The figure shows three views and two pictorial views of one solid part (mm, origin at its lowest corner). Answer the questions. Round coordinates to 2 decimals unless told otherwise and drop trailing zeros. Write each loop counter-clockwise with the first axis right and the second up, starting at its lowest first coordinate (ties: lowest second). Pieces come first, ordered by that corner, then holes.
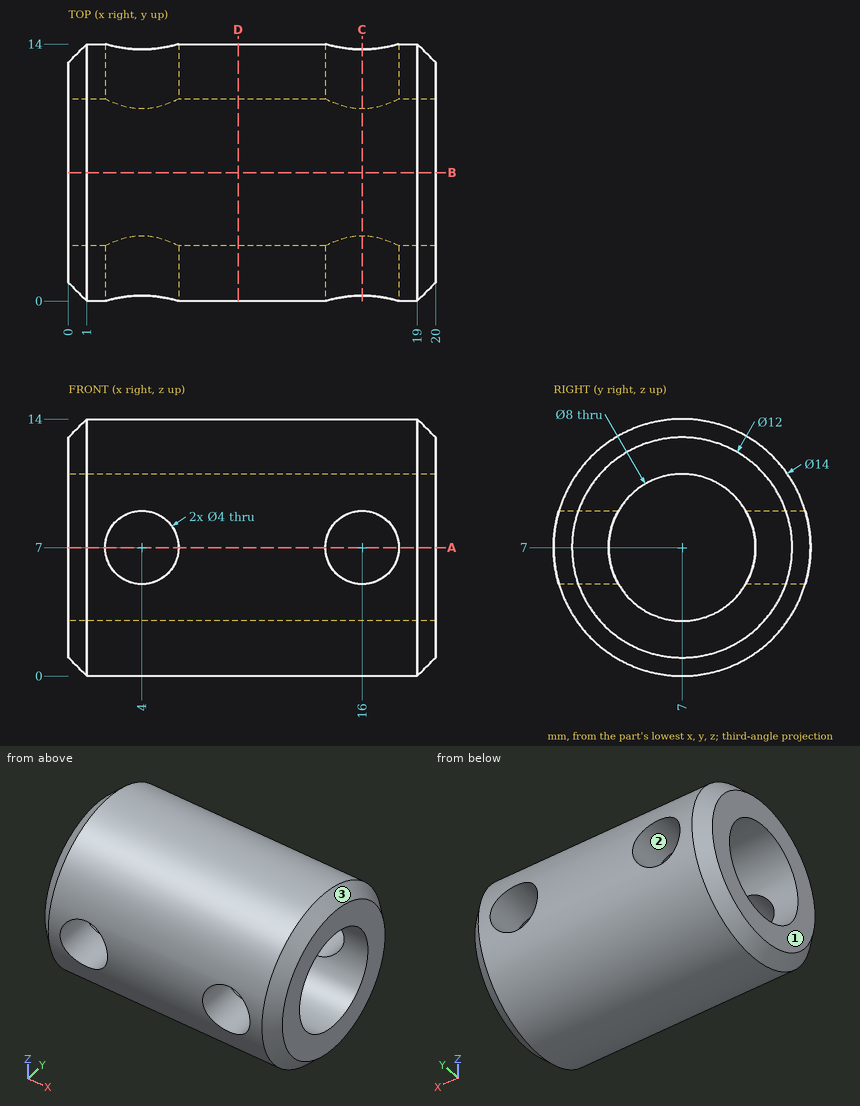
Q1. Section A-A (z = 7) is taken. Determine the outline of the cut face in (x, y).
Verdict:
outline: (0, 1) - (1, 0) - (2, 0) - (2, 3) - (0, 3) - close; (0, 11) - (2, 11) - (2, 14) - (1, 14) - (0, 13) - close; (6, 0) - (14, 0) - (14, 3) - (6, 3) - close; (6, 11) - (14, 11) - (14, 14) - (6, 14) - close; (18, 0) - (19, 0) - (20, 1) - (20, 3) - (18, 3) - close; (18, 11) - (20, 11) - (20, 13) - (19, 14) - (18, 14) - close
Q2. Flat-ended cylindrical pins translate along their axes: pin 1 Ø1.5 at (x, y) = (4.5, 8) entering from -Z; pin 2 Ø2 at (x, z) = (10, 12.5) entering from +Y; pin 3 Ø6 at (x, z) = (13, 11) entering from +Y. Find the tip coordinate at first contact, or state that the pin passes through.
Verdict:
pin 1: stops at z = 0
pin 2: stops at y = 12.36
pin 3: stops at y = 13.93
Q3. Straight lines are drawn through the part: probe 1 along X at (y, z) = (2.7, 7); probe 2 along X at (y, z) = (12.25, 5.75); probe 3 along Y at (x, z) = (10.5, 9). For each, find the intervals that lie inside material, in ascending order.
Verdict:
probe 1: x = 0 to 2, 6 to 14, 18 to 20
probe 2: x = 0 to 2.44, 5.56 to 14.44, 17.56 to 20
probe 3: y = 0.29 to 3.54, 10.46 to 13.71
Q4. Section D-D (x = 9.25) is taken. Determine the outline of the cut face in (y, z), then the cut area to 3 significant figures.
Verdict:
outline: circle Ø14 at (7, 7); hole circle Ø8 at (7, 7)
area: 104 mm2
Q5. Section C-C (x = 16) is taken. Determine the outline of the cut face in (y, z).
Verdict:
outline: (0.29, 5) arc R7 ccw to (13.71, 5) - (10.46, 5) arc R4 cw to (3.54, 5) - close; (0.29, 9) - (3.54, 9) arc R4 cw to (10.46, 9) - (13.71, 9) arc R7 ccw to start
Q6. Section B-B (y = 7) is taken. Determine the outline of the cut face in (x, z).
Verdict:
outline: (0, 1) - (1, 0) - (19, 0) - (20, 1) - (20, 3) - (0, 3) - close; (0, 11) - (20, 11) - (20, 13) - (19, 14) - (1, 14) - (0, 13) - close
Q7. Determine the mould class of the marked faces 1, 2 and 3 for opening direction X: pulls with the +X half, pulls with the -X half, needs draft (parallel to the pull), parting line crosses it, or undercut.
Verdict:
face 1: pulls with the -X half
face 2: undercut
face 3: pulls with the +X half
